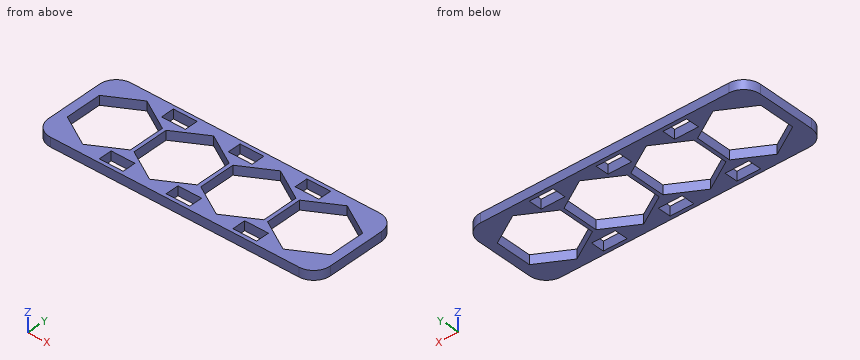
```python
from build123d import *

# Parameters (mm, degrees)
SKETCH1_W           = 8.128
SKETCH1_H           = 4.572
BOSS_EXTRUDE1_DEPTH = 3.175


with BuildPart() as part:
    # Sketch1 → Boss-Extrude1 (new body)
    with BuildSketch(Plane.XY):
        with BuildLine():
            Line((-8.255, 15.639992312), (76.835, 15.639992312))
            ThreePointArc((76.835, 15.639992312), (80.876115254, 13.966107566), (82.55, 9.924992312))
            Line((82.55, 9.924992312), (82.55, -9.924992312))
            ThreePointArc((82.55, -9.924992312), (80.876115254, -13.966107566), (76.835, -15.639992312))
            Line((76.835, -15.639992312), (-8.255, -15.639992312))
            ThreePointArc((-8.255, -15.639992312), (-12.296115254, -13.966107566), (-13.97, -9.924992312))
            Line((-13.97, -9.924992312), (-13.97, 9.924992312))
            ThreePointArc((-13.97, 9.924992312), (-12.296115254, 13.966107566), (-8.255, 15.639992312))
        make_face()
        Polygon((12.065, -6.232496156), (22.86, -12.464992312), (33.655, -6.232496156), (33.655, 6.232496156), (22.86, 12.464992312), (12.065, 6.232496156), align=None, mode=Mode.SUBTRACT)
        Polygon((34.925, -6.232496156), (45.72, -12.464992312), (56.515, -6.232496156), (56.515, 6.232496156), (45.72, 12.464992312), (34.925, 6.232496156), align=None, mode=Mode.SUBTRACT)
        Polygon((-10.795, -6.232496156), (0, -12.464992312), (10.795, -6.232496156), (10.795, 6.232496156), (0, 12.464992312), (-10.795, 6.232496156), align=None, mode=Mode.SUBTRACT)
        Polygon((57.785, -6.232496156), (68.58, -12.464992312), (79.375, -6.232496156), (79.375, 6.232496156), (68.58, 12.464992312), (57.785, 6.232496156), align=None, mode=Mode.SUBTRACT)
        with Locations((34.29, 12.083992312)):
            Rectangle(SKETCH1_W, SKETCH1_H, mode=Mode.SUBTRACT)
        with Locations((11.43, 12.083992312)):
            Rectangle(SKETCH1_W, SKETCH1_H, mode=Mode.SUBTRACT)
        with Locations((57.15, 12.083992312)):
            Rectangle(SKETCH1_W, SKETCH1_H, mode=Mode.SUBTRACT)
        with Locations((57.15, -12.083992312)):
            Rectangle(SKETCH1_W, SKETCH1_H, mode=Mode.SUBTRACT)
        with Locations((34.29, -12.083992312)):
            Rectangle(SKETCH1_W, SKETCH1_H, mode=Mode.SUBTRACT)
        with Locations((11.43, -12.083992312)):
            Rectangle(SKETCH1_W, SKETCH1_H, mode=Mode.SUBTRACT)
    extrude(amount=BOSS_EXTRUDE1_DEPTH)


solid = part.part
```
For this review, take the finished solid that the model builds, in its own axes (mm). Give positions to 0.01 mm unless a question says otherwise; leave off trailing zeros. Write each loop counter-clockwise with the first axis right and the second up, starting at its lowest first coordinate (ties: lowest second). Pieces come first, ordered by that corner, then holes.
Item 1: Insertion check: P1, Ø1, axis at y = -13, z = 1, coming from the +X side; P2, Ø1.6, axis at y = 12.5, z = 1, coming from the +X side; P3, Ø1.6, axis at y = -13, z = 1, coming from the +X side. Each pin has a flat end and moves straight along its axis. Give the tip position at first contact, or say it passes through.
Item 2: Wall thickness on probe 1 along X at (y, z) = (-4, 2) (3 decimals); probe 2 along Y at (x, z) = (11.5, 2.25); probe 3 along Y at (x, z) = (10, 2.55): over which ranges is each line inside the solid? List them lowest first.
Item 3: Take a section at A-A (y = 1). Give the boundary of the cut face in (x, z) (3 decimals).
Item 4: Take a section at D-D (x = 3.5). Give the boundary of the cut face in (y, z) (3 decimals).
Item 5: Take a section at C-C (y = 11.5). Give the number of separate pieces and of enclosed holes in the cut face, and give its area (3 significant figures).
Item 6: Take a section at B-B (x = 31.5). Give the boundary of the cut face in (y, z) (3 decimals), and give its area (3 significant figures).
Established:
1. P1: stops at x = 81.94
1. P2: stops at x = 82.27
1. P3: stops at x = 82.08
2. probe 1: x = -13.97 to -10.795, 10.795 to 12.065, 33.655 to 34.925, 56.515 to 57.785, 79.375 to 82.55
2. probe 2: y = -15.64 to -14.37, -9.8 to 9.8, 14.37 to 15.64
2. probe 3: y = -15.64 to -14.37, -9.8 to -6.69, 6.69 to 9.8, 14.37 to 15.64
3. outline: (-13.97, 0) - (-10.795, 0) - (-10.795, 3.175) - (-13.97, 3.175) - close; (10.795, 0) - (12.065, 0) - (12.065, 3.175) - (10.795, 3.175) - close; (33.655, 0) - (34.925, 0) - (34.925, 3.175) - (33.655, 3.175) - close; (56.515, 0) - (57.785, 0) - (57.785, 3.175) - (56.515, 3.175) - close; (79.375, 0) - (82.55, 0) - (82.55, 3.175) - (79.375, 3.175) - close
4. outline: (-15.64, 0) - (-10.444, 0) - (-10.444, 3.175) - (-15.64, 3.175) - close; (10.444, 0) - (15.64, 0) - (15.64, 3.175) - (10.444, 3.175) - close
5. separate pieces: 8
5. enclosed holes: 0
5. area: 185 mm2
6. outline: (-15.64, 0) - (-14.37, 0) - (-14.37, 3.175) - (-15.64, 3.175) - close; (-9.798, 0) - (-7.477, 0) - (-7.477, 3.175) - (-9.798, 3.175) - close; (7.477, 0) - (9.798, 0) - (9.798, 3.175) - (7.477, 3.175) - close; (14.37, 0) - (15.64, 0) - (15.64, 3.175) - (14.37, 3.175) - close
6. area: 22.8 mm2
